Design review of the part built by this model. Coordinates are the model's own, in mm. Give positions to 0.01 mm unless a question says otherwise; leave off trailing zeros. Loops run counter-clockwise (first coordinate to the right, second up) from the corner with the lowest first, then second, coordinate; pieces in that order, holes last. Notation, with made-up numbers: (29.5, 22) -> (35.5, 22) arc R16 cw to (35.5, 38) -> close; hole circle Ø4 at (-32.75, -25.75). An arc over 180 degrees is marked (long way). Use CSV: the item, a comma, the result in double quotes. Start each with the question number.
Item 1: We need section B-B (x = 8.75). State the section outline as (y, z) points.
Item 2: We need section A-A (z = 1.7). State the section outline as (x, y) points.
Item 3: Wall thickness on line 1 along X through (y, z) = (9, 1.2); line 2 along Y through (x, z) = (8.5, -0.05); line 3 along Y through (x, z) = (9.25, -0.85): over which ranges is each line inside the solid? List them lowest first. Write a range as from..to.
from build123d import *

# Parameters (mm, degrees)
SKETCH1_W           = 20
SKETCH1_H           = 20
BOSS_EXTRUDE1_DEPTH = 2.5
FILLET1_R           = 3


with BuildPart() as part:
    # Sketch1 → Boss-Extrude1 (new, symmetric)
    with BuildSketch(Plane.XY):
        Rectangle(SKETCH1_W, SKETCH1_H)
    extrude(amount=BOSS_EXTRUDE1_DEPTH, both=True)

    # Fillet1
    fillet1_edges = [part.edges().sort_by_distance(p)[0] for p in [
        (10, -10, 0),
        (-10, -10, 0),
        (-10, 10, 0),
        (10, 10, 0),
    ]]
    fillet(fillet1_edges, radius=FILLET1_R)


solid = part.part
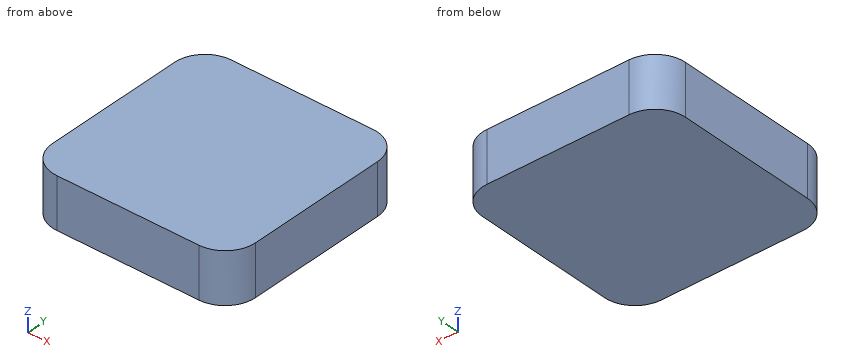
Results found:
1,outline,"(-9.44, -2.5) -> (9.44, -2.5) -> (9.44, 2.5) -> (-9.44, 2.5) -> close"
2,outline,"(-10, -7) arc R3 ccw to (-7, -10) -> (7, -10) arc R3 ccw to (10, -7) -> (10, 7) arc R3 ccw to (7, 10) -> (-7, 10) arc R3 ccw to (-10, 7) -> close"
3,line 1,"-9.24..9.24"
3,line 2,"-9.6..9.6"
3,line 3,"-8.98..8.98"
